Source: CAD feature listing. Evaluate the final solid. Frame: model axes, mm. Face numbers are marked on the shaded views. A direction names the side the tool comes from. Give positions to 0.01 mm unless a question says otherwise; leave off trailing zeros. Order: outer loops, then holes, each group sorted by start corner. A loop starts at its lowest first (then second) coordinate and runs counter-clockwise, first axis right, second up. Notation, with made-up numbers: M 6.5,26 L 62.5,26 A16 ccw 62.5,57 Z; hole C 48,-31 d3. An arc over 180 degrees is marked long. Use CSV: the item, a comma, the result in double quotes. Start each with the question number.
1. Section query A-A, the plane y = 17.5. Return the cut outline in (x, z).
2. Mould query, pull axis X, two halves, no side actions, for the marked faces 1, 2 and 3. Classes: released by +X, released by -X, zero draft, split by the parting line, or undercut.
3. Reachability of the marked faces 4, 5, 6, 7 and 8 from +Z, -Z, +X, -X, +Y, -Y: full face, straight path, thin tool, end or side. Return the list, or none.
4. Section query B-B, the plane z = 1. Return the cut outline in (x, y).
5. Line query: line 1 along Z through (x, y) = (6.5, 18.25); line 2 along X through (y, z) = (9.75, 3.75); line 3 along Y through (x, z) = (-3.25, 0.25). Output: solid intervals per line, ascending. Write a range as [from, to].
6. Pin query (flat end, axial travel): P1, Ø0.5, axis at y = 11.5, z = 4, coming from the +X side; P2, Ø0.8, axis at x = 4.5, z = 4, coming from the -Y side; P3, Ø3, axis at x = 0, z = 0, coming from the +Y side. Return the tip coordinate at first contact, or that it passes through.
7. Section query C-C, the plane y = 10. Return the cut outline in (x, z).
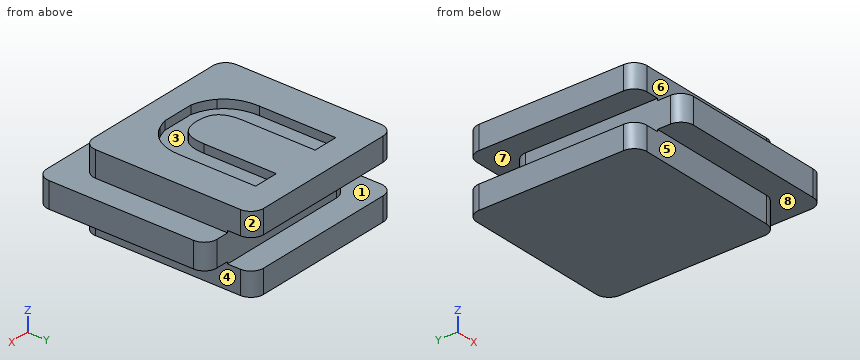
from build123d import *

# Parameters (mm, degrees)
F0_W     = 14
F0_H     = 3
F0_W_2   = 3
F1_DEPTH = 20
F2_DEPTH = 3
F3_W     = 3
F3_H     = 3
F4_DEPTH = 100
F5_W     = 3
F5_H     = 3.5
F6_DEPTH = 100
F7_R     = 1.5
F9_DEPTH = 1


with BuildPart() as f1:
    # F0 (on Front) → F1 (new body)
    with BuildSketch(Plane.XZ):
        Polygon((10, 1.5), (10, 4.5), (-10, 4.5), (-10, 1.5), (-7, 1.5), (7, 1.5), align=None)
        Rectangle(F0_W, F0_H)
        with Locations((11.5, 0)):
            Rectangle(F0_W_2, F0_H)
        with Locations((8.5, 0)):
            Rectangle(F0_W_2, F0_H)
        with Locations((-8.5, 0)):
            Rectangle(F0_W_2, F0_H)
        Polygon((10, -4.5), (10, -1.5), (7, -1.5), (-7, -1.5), (-10, -1.5), (-10, -4.5), align=None)
    extrude(amount=-F1_DEPTH)

    # F0 (on Front) → F2 (join)
    with BuildSketch(Plane.XZ):
        with Locations((-8.5, 0)):
            Rectangle(F0_W_2, F0_H)
        Rectangle(F0_W, F0_H)
        with Locations((8.5, 0)):
            Rectangle(F0_W_2, F0_H)
        with Locations((11.5, 0)):
            Rectangle(F0_W_2, F0_H)
    extrude(amount=F2_DEPTH)

    # F3 (on face) → F4 (cut)
    with BuildSketch(Plane.YZ.offset(13)):
        Polygon((23, -1.75), (23, 1.75), (17, 1.75), (17, 1.5), (20, 1.5), (20, -1.5), (17, -1.5), (17, -1.75), align=None)
        with Locations((18.5, 0)):
            Rectangle(F3_W, F3_H)
    extrude(amount=-F4_DEPTH, mode=Mode.SUBTRACT)

    # F5 (on face) → F6 (cut)
    with BuildSketch(Plane(origin=(0, 17, 0), x_dir=(-1, 0, 0), z_dir=(0, 1, 0))):
        with Locations((11.5, 0)):
            Rectangle(F5_W, F5_H)
        with Locations((8.5, 0)):
            Rectangle(F5_W, F5_H)
    extrude(amount=-F6_DEPTH, mode=Mode.SUBTRACT)

    # F7
    f7_edges = [f1.edges().sort_by_distance(p)[0] for p in [
        (-7, -3, 0),
        (13, -3, 0),
        (10, 0, 3),
        (10, 0, -3),
        (-10, 0, -3.125),
        (-10, 0, 3.125),
        (-7, 17, 0),
        (-10, 20, 3.125),
        (-10, 20, -3.125),
        (13, 17, 0),
        (10, 20, 3.125),
        (10, 20, -3.125),
    ]]
    fillet(f7_edges, radius=F7_R)

    # F8 (on face) → F9 (cut)
    with BuildSketch(Plane.XY.offset(4.5)):
        with BuildLine():
            Line((-1.7204794807, 3), (1.9396642309, 3))
            add(Edge.make_bspline(
                [(3.1876434099, 3.4268663194), (2.6101370894, 3.1526013575), (1.9396642309, 3)],
                knots=[0, 0, 0, 0.4435987872, 0.4435987872, 0.4435987872], degree=2))
            add(Edge.make_bspline(
                [(5.177660771, 5.2026909722), (4.4895097293, 4.0451388889), (3.1876434099, 3.4268663194)],
                knots=[0, 0, 0, 1, 1, 1], degree=2))
            add(Edge.make_bspline(
                [(5.8658118126, 7.9006076389), (5.8658118126, 6.3602430556), (5.177660771, 5.2026909722)],
                knots=[0, 0, 0, 1, 1, 1], degree=2))
            Line((5.8658118126, 7.9006076389), (5.8658118126, 16.8815104167))
            Line((5.8658118126, 16.8815104167), (2.9309159793, 16.8815104167))
            Line((2.9309159793, 16.8815104167), (2.9309159793, 8.4019097222))
            add(Edge.make_bspline(
                [(2.2807423682, 6.0336371528), (2.9309159793, 6.7886284722), (2.9309159793, 8.4019097222)],
                knots=[0, 0, 0, 1, 1, 1], degree=2))
            add(Edge.make_bspline(
                [(0.187426396, 5.2786458333), (1.6305687571, 5.2786458333), (2.2807423682, 6.0336371528)],
                knots=[0, 0, 0, 1, 1, 1], degree=2))
            add(Edge.make_bspline(
                [(-1.9499433957, 6.0290798611), (-1.3043270763, 5.2786458333), (0.187426396, 5.2786458333)],
                knots=[0, 0, 0, 1, 1, 1], degree=2))
            add(Edge.make_bspline(
                [(-2.5955597151, 8.3836805556), (-2.5955597151, 6.7795138889), (-1.9499433957, 6.0290798611)],
                knots=[0, 0, 0, 1, 1, 1], degree=2))
            Line((-2.5955597151, 8.3836805556), (-2.5955597151, 16.8815104167))
            Line((-2.5955597151, 16.8815104167), (-5.527417354, 16.8815104167))
            Line((-5.527417354, 16.8815104167), (-5.527417354, 7.9370659722))
            add(Edge.make_bspline(
                [(-4.0462975624, 4.1818576389), (-5.527417354, 5.5551215278), (-5.527417354, 7.9370659722)],
                knots=[0, 0, 0, 1, 1, 1], degree=2))
            add(Edge.make_bspline(
                [(-1.7204794807, 3), (-3.1181346209, 3.3212839988), (-4.0462975624, 4.1818576389)],
                knots=[0.3733370206, 0.3733370206, 0.3733370206, 1, 1, 1], degree=2))
        make_face()
    extrude(amount=-F9_DEPTH, mode=Mode.SUBTRACT)


solid = f1.part
Result set:
1,outline,"M -10,-4.5 L 10,-4.5 L 10,-1.75 L -10,-1.75 Z; M -10,1.75 L 10,1.75 L 10,4.5 L -10,4.5 Z"
2,face 1,"zero draft"
2,face 2,"released by +X"
2,face 3,"undercut"
3,face 4,"-Z, +X, +Y, -Y"
3,face 5,"-Z, +X, -X, -Y"
3,face 6,"+Z, +X, -X, -Y"
3,face 7,"-X, +Y"
3,face 8,"-Z, +X, -Y"
4,outline,"M -7,-1.5 A1.5 ccw -5.5,-3 L 11.5,-3 A1.5 ccw 13,-1.5 L 13,15.5 A1.5 ccw 11.5,17 L -5.5,17 A1.5 ccw -7,15.5 Z"
5,line 1,"[-4.5, -1.75], [1.75, 4.5]"
5,line 2,"[-10, -5.53], [-2.6, 2.93], [5.87, 10]"
5,line 3,"[-3, 17]"
6,P1,"x = 10"
6,P2,"y = 0"
6,P3,"y = 17"
7,outline,"M -10,-4.5 L 10,-4.5 L 10,-1.5 L 13,-1.5 L 13,1.5 L 10,1.5 L 10,4.5 L 5.87,4.5 L 5.87,3.5 L 2.93,3.5 L 2.93,4.5 L -2.6,4.5 L -2.6,3.5 L -5.53,3.5 L -5.53,4.5 L -10,4.5 L -10,1.75 L -7,1.75 L -7,-1.75 L -10,-1.75 Z"
